from build123d import *

# Parameters (mm, degrees)
BOSS_EXTRUDE1_DEPTH = 6.35
SKETCH3_W           = 12.7
SKETCH3_H           = 6.35
BOSS_EXTRUDE2_DEPTH = 19.05
SKETCH4_R           = 5
CUT_EXTRUDE1_DEPTH  = 12.7
LPATTERN1_COUNT     = 2
LPATTERN1_PITCH     = 40.64
SKETCH5_R           = 5.5
BOSS_EXTRUDE3_DEPTH = 19.05
SKETCH10_R          = 7.62
BOSS_EXTRUDE4_DEPTH = 1.5


with BuildPart() as part:
    # Sketch2 → Boss-Extrude1 (new body)
    with BuildSketch(Plane(origin=(0, 0, 0), x_dir=(1, 0, 0), z_dir=(0, 1, 0))):
        Polygon((-38.1, 0), (38.1, 0), (38.1, 50.8), (19.05, 63.5), (-19.05, 63.5), (-38.1, 50.8), align=None)
    extrude(amount=BOSS_EXTRUDE1_DEPTH)

    # Sketch3 → Boss-Extrude2 (add)
    with BuildSketch(Plane(origin=(0, 6.35, 0), x_dir=(1, 0, 0), z_dir=(0, 1, 0))):
        with Locations((-0.072298758, 4.346211763)):
            Rectangle(SKETCH3_W, SKETCH3_H)
    boss_extrude2 = extrude(amount=BOSS_EXTRUDE2_DEPTH)

    # Sketch4 → Cut-Extrude1 (cut)
    with BuildSketch(Plane.XY.offset(-1.171211763)):
        with Locations((-0.072298758, 13.524669763)):
            Circle(SKETCH4_R)
    cut_extrude1 = extrude(amount=-CUT_EXTRUDE1_DEPTH, mode=Mode.SUBTRACT)

    # LPattern1: Boss-Extrude2, Cut-Extrude1 ×2
    with Locations(*[(0, 0, -i * LPATTERN1_PITCH) for i in range(1, LPATTERN1_COUNT)]):
        add(boss_extrude2)
        add(cut_extrude1, mode=Mode.SUBTRACT)

    # Sketch5 → Boss-Extrude3 (add)
    with BuildSketch(Plane(origin=(0, 6.35, 0), x_dir=(1, 0, 0), z_dir=(0, 1, 0))):
        with Locations((-26.317835068, 24.666211763)):
            Circle(SKETCH5_R)
        with Locations((26.173237553, 24.666211763)):
            Circle(SKETCH5_R)
    extrude(amount=BOSS_EXTRUDE3_DEPTH)

    # Sketch10 → Boss-Extrude4 (add)
    with BuildSketch(Plane(origin=(0, 6.35, 0), x_dir=(1, 0, 0), z_dir=(0, 1, 0))):
        with Locations((-26.31783504, 24.666211763)):
            Circle(SKETCH10_R)
        with Locations((26.173237524, 24.666211763)):
            Circle(SKETCH10_R)
    extrude(amount=BOSS_EXTRUDE4_DEPTH)


solid = part.part
CAD build for the part. Positions are in the model's coordinates, mm. A direction names the side the tool comes from. Round coordinates to 2 decimals unless told otherwise and drop trailing zeros. Write each loop counter-clockwise with the first axis right and the second up, starting at its lowest first coordinate (ties: lowest second). Pieces come first, ordered by that corner, then holes. Notation, with made-up numbers: M -35.5,76 L -30.5,76 A9 ccw -30.5,85 Z; hole C -19,-25 d3. An arc over 180 degrees is marked long. Put each result on its own line as item: value. Start each with the question number.
1) Saw through at C-C, the plane x = 25.5. Write the cut outline in (y, z).
2) Saw through at B-B, the plane y = 23.5. Write the cut outline in (x, z), and give its area (3 significant figures).
3) Pull direction Y, two halves, no side cores. Call faces 6 (the cylindrical face through (-1.156, 8.644, -44.942)), 7 (the flat face through (0, 25.4, -4)), 8 (the flat face through (-3, 18, -1.171)): pulls with the +Y half, pulls with the -Y half, needs draft (parallel to the pull), parting line crosses it, or undercut.
4) Saw through at D-D, the plane z = -6.5. Write the cut outline in (x, y), and give its area (3 significant figures).
5) Pin check, flat tips, straight feed: pin 1 Ø1.5 at (y, z) = (15.5, -31.5) entering from +X; pin 2 Ø3 at (x, z) = (23, -32.5) entering from -Y; pin 3 Ø7 at (y, z) = (15, -3.5) entering from -X; pin 4 Ø10 at (x, y) = (1, 14.5) entering from -Z. Stop position of each tip, or through.
6) Drill centre lines: probe 1 along Z at (x, y) = (-4.5, 10.5); probe 2 along Y at (x, z) = (-24, -17.5); probe 3 along Y at (x, z) = (28, -41). Where is each one in solid material? Low to high. Write a range as [from, to].
7) 3-axis set-ups, long thin cutter, end or side, ignore diameter. For faces 1 (the flat face through (-3, 18, -41.811)), 2 (the flat face through (6.278, 16, -4)), 3 (the flat face through (-1, 0, -32)), 4 (the flat face through (0, 3, -63.5)), 5 (the cylindrical face through (20.126, 7.089, -20.03)): which of +Z, -Z, +X, -X, +Y, -Y reach the whole face in a straight line?
8) Saw through at A-A, the plane y = 10.75. Write the cut outline in (x, z).
Resolved:
1. outline: M 0,-59.2 L 6.35,-59.2 L 6.35,-32.26 L 7.85,-32.26 L 7.85,-30.12 L 25.4,-30.12 L 25.4,-19.21 L 7.85,-19.21 L 7.85,-17.08 L 6.35,-17.08 L 6.35,0 L 0,0 Z
2. outline: C -26.32,-24.67 d11; M -6.42,-48.16 L 6.28,-48.16 L 6.28,-41.81 L -6.42,-41.81 Z; M -6.42,-7.52 L 6.28,-7.52 L 6.28,-1.17 L -6.42,-1.17 Z; C 26.17,-24.67 d11
2. area: 351 mm²
3. face 6: undercut
3. face 7: pulls with the +Y half
3. face 8: needs draft
4. outline: M -38.1,0 L 38.1,0 L 38.1,6.35 L 6.28,6.35 L 6.28,25.4 L -6.42,25.4 L -6.42,6.35 L -38.1,6.35 Z; hole C -0.07,13.52 d10
4. area: 647 mm²
5. pin 1: through
5. pin 2: y = 0
5. pin 3: x = -6.42
5. pin 4: z = -48.16
6. probe 1: [-48.16, -41.81], [-7.52, -1.17]
6. probe 2: [0, 7.85]
6. probe 3: [0, 6.35]
7. face 1: +X, -X, +Y
7. face 2: +Z, -Z, +X, +Y
7. face 3: +Z, -Z, +X, -X, -Y
7. face 4: -Z, +X, -X, +Y, -Y
7. face 5: +Y
8. outline: C -26.32,-24.67 d11; M -6.42,-48.16 L -4.23,-48.16 L -4.23,-41.81 L -6.42,-41.81 Z; M -6.42,-7.52 L -4.23,-7.52 L -4.23,-1.17 L -6.42,-1.17 Z; M 4.09,-48.16 L 6.28,-48.16 L 6.28,-41.81 L 4.09,-41.81 Z; M 4.09,-7.52 L 6.28,-7.52 L 6.28,-1.17 L 4.09,-1.17 Z; C 26.17,-24.67 d11
